```python
from build123d import *

# Parameters (mm, degrees)
SCHIZZO1_R                      = 5
ESTRUSIONE_ESTRUSIONE1_DEPTH    = 14
SCHIZZO2_R                      = 3
ESTRUSIONE_ESTRUSIONE2_DEPTH    = 2
FORO_FILETTATO_M6_1_D           = 5
FORO_FILETTATO_M6_1_DEPTH       = 6
FORO_FILETTATO_M6_1_CSINK_D     = 7
FORO_FILETTATO_M6_1_CSINK_ANGLE = 90
FORO_FILETTATO_M6_1_TIP         = 1.502151548


with BuildPart() as part:
    # Schizzo1 → Estrusione-Estrusione1 (new body)
    with BuildSketch(Plane.XY):
        Circle(SCHIZZO1_R)
    extrude(amount=ESTRUSIONE_ESTRUSIONE1_DEPTH)

    # Schizzo2 → Estrusione-Estrusione2 (add)
    with BuildSketch(Plane.XY.offset(14)):
        Circle(SCHIZZO2_R)
    extrude(amount=ESTRUSIONE_ESTRUSIONE2_DEPTH)

    # Foro filettato M6-1
    with Locations(Plane(origin=(0, 0, 0), x_dir=(-1, 0, 0), z_dir=(0, 0, -1))):
        with Locations((0, 0)):
            CounterSinkHole(FORO_FILETTATO_M6_1_D / 2, FORO_FILETTATO_M6_1_CSINK_D / 2, depth=FORO_FILETTATO_M6_1_DEPTH, counter_sink_angle=FORO_FILETTATO_M6_1_CSINK_ANGLE)
            with Locations((0, 0, -(FORO_FILETTATO_M6_1_DEPTH + FORO_FILETTATO_M6_1_TIP / 2))):  # 118° drill point
                Cone(0, FORO_FILETTATO_M6_1_D / 2, FORO_FILETTATO_M6_1_TIP, mode=Mode.SUBTRACT)


solid = part.part
```
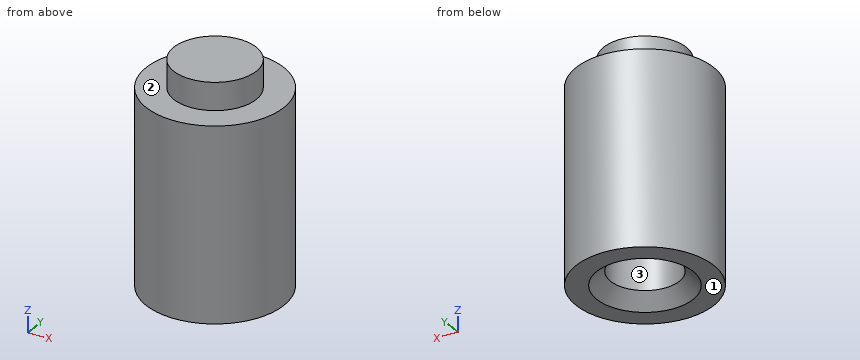
Geometry: final body of the model. Coordinates: model frame, mm. Face numbers are marked on the shaded views. A direction names the side the tool comes from. Coordinates: 2 decimals unless noted, no trailing zeros. Order: outer loops, then holes, each group sorted by start corner. A loop starts at its lowest first (then second) coordinate and runs counter-clockwise, first axis right, second up. Notation, with made-up numbers: (15, 32.5) -> (45, 32.5) arc R34 cw to (45, 65.5) -> close; hole circle Ø4 at (23.5, 19). An arc over 180 degrees is marked (long way). Answer in a Markdown table with one row per item.
Item 1: Ray query, L1, parallel to Y at x = 0, z = 4.4; L2, parallel to Z at x = 0, y = 4.25; L3, parallel to X at y = -2, z = 4. Return the intervals inside material, ascending.
Return value:
| item | result |
|---|---|
| L1 | y = -5 to -2.5, 2.5 to 5 |
| L2 | z = 0 to 14 |
| L3 | x = -4.58 to -1.5, 1.5 to 4.58 |
Item 2: Section B-B on z = 7. Output: boundary loops of the cut face in (x, y).
Return value:
| item | result |
|---|---|
| outline | circle Ø10 at (0, 0); hole circle Ø1.67 at (0, 0) |
Item 3: Access query for the marked faces 1, 2 and 3. Directions: +Z, -Z, +X, -X, +Y, -Y. A direction counts if a zero-diameter tool reaches every point of the face in a straight line with its end or side. Return the directions, or none.
Return value:
| item | result |
|---|---|
| face 1 | -Z, +X, -X, +Y, -Y |
| face 2 | +Z |
| face 3 | -Z |
Item 4: Section C-C on y = 3.75. Output: boundary loops of the cut face in (x, z), plus the area to 3 significant figures.
Return value:
| item | result |
|---|---|
| outline | (-3.31, 0) -> (3.31, 0) -> (3.31, 14) -> (-3.31, 14) -> close |
| area | 92.6 mm² |
Item 5: Section A-A on z = 9.75. Output: boundary loops of the cut face in (x, y), plus the area to 3 significant figures.
Return value:
| item | result |
|---|---|
| outline | circle Ø10 at (0, 0) |
| area | 78.5 mm² |
Item 6: Contact query for flat-ended pins moving along their axis: P1, Ø2, axis at x = -4, y = -2, coming from the -Z side; P2, Ø1, axis at y = 1, z = 5, coming from the -X side; P3, Ø2, axis at x = 2.5, z = 12, coming from the -Y side; P4, Ø5, axis at x = -3, z = 7.5, coming from the +Y side. Output: stop coordinate, or through.
Return value:
| item | result |
|---|---|
| P1 | stops at z = 0 |
| P2 | stops at x = -4.97 |
| P3 | stops at y = -4.77 |
| P4 | stops at y = 4.97 |
